from build123d import *

# Parameters (mm, degrees)
SKETCH1_R           = 21
BOSS_EXTRUDE1_DEPTH = 6
SKETCH2_R           = 10.5
BOSS_EXTRUDE2_DEPTH = 24
SKETCH3_R           = 6
CUT_EXTRUDE1_DEPTH  = 43.213741838
SKETCH4_R           = 2.25
CUT_EXTRUDE2_DEPTH  = 39.183766184


with BuildPart() as part:
    # Sketch1 → Boss-Extrude1 (new body)
    with BuildSketch(Plane.XY):
        Circle(SKETCH1_R)
    extrude(amount=BOSS_EXTRUDE1_DEPTH)

    # Sketch2 → Boss-Extrude2 (add)
    with BuildSketch(Plane.XY.offset(6)):
        Circle(SKETCH2_R)
    extrude(amount=BOSS_EXTRUDE2_DEPTH)

    # Sketch3 → Cut-Extrude1 (cut, through all)
    with BuildSketch(Plane.XY.offset(30)):
        Circle(SKETCH3_R)
    extrude(amount=-CUT_EXTRUDE1_DEPTH, mode=Mode.SUBTRACT)

    # Sketch4 → Cut-Extrude2 (cut, through all)
    with BuildSketch(Plane.XY.offset(6)):
        with Locations((-16, 0)):
            Circle(SKETCH4_R)
        with Locations((0, 16)):
            Circle(SKETCH4_R)
        with Locations((16, 0)):
            Circle(SKETCH4_R)
        with Locations((0, -16)):
            Circle(SKETCH4_R)
    extrude(amount=-CUT_EXTRUDE2_DEPTH, mode=Mode.SUBTRACT)


solid = part.part
Work out the finished part from the listing and answer in its coordinate system (mm). A direction names the side the tool comes from. Give positions to 0.01 mm unless a question says otherwise; leave off trailing zeros. Loops run counter-clockwise (first coordinate to the right, second up) from the corner with the lowest first, then second, coordinate; pieces in that order, holes last. Notation, with made-up numbers: (56, 86) - (86, 86) arc R31 cw to (86, 113) - close; hole circle Ø1 at (15.5, -31.5). An arc over 180 degrees is marked (long way). Answer in a Markdown table with one row per item. Add a question column.
Q1. Consider line 1 along Y through (x, z) = (0, 4.65); line 2 along Y through (x, z) = (0, 20.5); line 3 along Z through (x, y) = (-3, -17.5). Determine where each line is inside the solid, lowest interval first.
Q2. Each of these flat-tipped pins is pushed along its axis until it touches: P1, Ø4, axis at y = 1.5, z = 19.5, coming from the -X side; P2, Ø5, axis at x = 0, y = 16, coming from the +Z side; P3, Ø2, axis at y = -16, z = 6, coming from the +X side. Where does it stop, or does it pass through?
Q3. Determine the mould class of faces 1 (the flat face through (5, -5, 30)), 2 (the cylindrical face through (20.03, 6.31, 2.96)), 3 (the cylindrical face through (-6, 0, 15)) for opening direction Y: released by +Y, released by -Y, zero draft, split by the parting line, or undercut.
Q4. The part is cut by section D-D (y = 14.5). Determine the outline of the cut face in (x, z), and give its area (3 significant figures).
Q5. A tool of negligible diameter and unlimited length cuts with its end or side. For faces 4 (the cylindrical face through (-0.488, -18.196, 3.042)), 5 (the cylindrical face through (10, 3.2, 17.8)), from which of +Z, -Z, +X, -X, +Y, -Y can it reach the whole face along a straight path? Write none if from no direction.
Q6. The part is cut by section A-A (x = 0). Determine the outline of the cut face in (y, z), and give its area (3 significant figures).
Q7. The part is cut by section C-C (z = 2.25). Determine the outline of the cut face in (x, y), and give its area (3 significant figures).
Solution:
| question | item | result |
|---|---|---|
| 1 | line 1 | y = -21 to -18.25, -13.75 to -6, 6 to 13.75, 18.25 to 21 |
| 1 | line 2 | y = -10.5 to -6, 6 to 10.5 |
| 1 | line 3 | z = 0 to 6 |
| 2 | P1 | stops at x = -10.5 |
| 2 | P2 | stops at z = 6 |
| 2 | P3 | stops at x = 14.7 |
| 3 | face 1 | zero draft |
| 3 | face 2 | split by the parting line |
| 3 | face 3 | undercut |
| 4 | outline | (-15.19, 0) - (-1.68, 0) - (-1.68, 6) - (-15.19, 6) - close; (1.68, 0) - (15.19, 0) - (15.19, 6) - (1.68, 6) - close |
| 4 | area | 162 mm² |
| 5 | face 4 | +Z, -Z |
| 5 | face 5 | +Z |
| 6 | outline | (-21, 0) - (-18.25, 0) - (-18.25, 6) - (-21, 6) - close; (-13.75, 0) - (-6, 0) - (-6, 30) - (-10.5, 30) - (-10.5, 6) - (-13.75, 6) - close; (6, 0) - (13.75, 0) - (13.75, 6) - (10.5, 6) - (10.5, 30) - (6, 30) - close; (18.25, 0) - (21, 0) - (21, 6) - (18.25, 6) - close |
| 6 | area | 342 mm² |
| 7 | outline | circle Ø42 at (0, 0); hole circle Ø4.5 at (-16, 0); hole circle Ø12 at (0, 0); hole circle Ø4.5 at (0, -16); hole circle Ø4.5 at (0, 16); hole circle Ø4.5 at (16, 0) |
| 7 | area | 1,210 mm² |
